from build123d import *

# Parameters (mm, degrees)
BOSS_EXTRUDE1_DEPTH = 2
CUT_EXTRUDE2_DEPTH  = 2
SKETCH5_R           = 2.25
CUT_EXTRUDE4_DEPTH  = 2


with BuildPart() as part:
    # Sketch1 → Boss-Extrude1 (new body)
    with BuildSketch(Plane(origin=(0, 0, 0), x_dir=(1, 0, 0), z_dir=(0, 1, 0))):
        Polygon((-14, -27.5), (-9, -27.5), (-9, -29.5), (-5, -29.5), (-5, -27.5), (5, -27.5), (5, -29.5), (9, -29.5), (9, -27.5), (14, -27.5), (14, 27.5), (9, 27.5), (9, 29.5), (5, 29.5), (5, 27.5), (-5, 27.5), (-5, 29.5), (-9, 29.5), (-9, 27.5), (-14, 27.5), (-14, 14.5), (-14, -14.5), align=None)
    extrude(amount=BOSS_EXTRUDE1_DEPTH)

    # Sketch4 → Cut-Extrude2 (cut)
    with BuildSketch(Plane(origin=(0, 2, 0), x_dir=(1, 0, 0), z_dir=(0, 1, 0))):
        Polygon((-1.5, 23.2), (-2.6, 23.2), (-2.6, 25.5), (-1.5, 25.5), (-1.5, 27.5), (1.5, 27.5), (1.5, 25.5), (2.6, 25.5), (2.6, 23.2), (1.5, 23.2), (1.5, 21.5), (-1.5, 21.5), align=None)
        Polygon((1.5, -25.5), (1.5, -27.5), (-1.5, -27.5), (-1.5, -25.5), (-2.6, -25.5), (-2.6, -23.2), (-1.5, -23.2), (-1.5, -21.5), (1.5, -21.5), (1.5, -23.2), (2.6, -23.2), (2.6, -25.5), align=None)
    extrude(amount=-CUT_EXTRUDE2_DEPTH, mode=Mode.SUBTRACT)

    # Sketch5 → Cut-Extrude4 (cut)
    with BuildSketch(Plane(origin=(0, 2, 0), x_dir=(1, 0, 0), z_dir=(0, 1, 0))):
        with Locations(Location((0, -9.51, 0), (0, 0, 270))):
            Circle(SKETCH5_R)
    extrude(amount=-CUT_EXTRUDE4_DEPTH, mode=Mode.SUBTRACT)


solid = part.part
Could you check a few things on this model? Use its own coordinates, in mm. A direction names the side the tool comes from. Give positions to 0.01 mm unless a question says otherwise; leave off trailing zeros. Write each loop counter-clockwise with the first axis right and the second up, starting at its lowest first coordinate (ties: lowest second). Pieces come first, ordered by that corner, then holes. Notation, with made-up numbers: (35, 20) - (75, 20) arc R23 cw to (75, 38) - close; hole circle Ø6 at (-15, 84). An arc over 180 degrees is marked (long way). Use CSV: the item, a comma, the result in double quotes. Start each with the question number.
Item 1: I want a section at A-A, the plane z = 9.51. Please give me the cut outline in (x, y), then the cut area to 3 significant figures.
Item 2: If we mould it in two halves opening along Z, with no side actions, what happens to faces 5 (the face through (0, 1, -21.5)), 6 (the face through (11, 1, 27.5)), 7 (the face through (0, 0, 0)), 8 (the face through (2, 1, -23.2))? For each: pulls with the +Z half, pulls with the -Z half, needs draft (parallel to the pull), parting line crosses it, or undercut.
Item 3: For faces 1 (the face through (-2.6, 1, 24)), 2 (the face through (-11, 1, -27.5)), 3 (the face through (-1.5, 1, -26)), 4 (the face through (1.5, 1, 22)), which set-ups out of +Z, -Z, +X, -X, +Y, -Y let a thin tool reach every point of the face, with its end or its side?
Item 4: I want a section at C-C, the plane x = -3.25. Please give me the cut outline in (y, z), then the cut area to 3 significant figures.
Item 5: If I drill on line 1 along X through (y, z) = (1.4, 27); line 2 along X through (y, z) = (0.9, 9.51); line 3 along Z through (x, y) = (-10.5, 0.95), over which ranges is the centre line in solid material (lowest first)?
Item 6: I want a section at B-B, the plane x = 0. Please give me the cut outline in (y, z).
Item 7: I'm going to push flat-ended pins straight in: pin 1 (7 mm diameter, centred on x = 0, z = 9.51, fed in from -Y); pin 2 (0.6 mm diameter, centred on x = 3, y = 0.5, fed in from +Z); pin 3 (1 mm diameter, centred on y = 1, z = 29, fed in from -X); pin 4 (1 mm diameter, centred on x = 0, y = 0.5, fed in from +Z). Where does each tip first touch, or does it pass through?
Findings:
1,outline,"(-14, 0) - (-2.25, 0) - (-2.25, 2) - (-14, 2) - close; (2.25, 0) - (14, 0) - (14, 2) - (2.25, 2) - close"
1,area,"47.0 mm2"
2,face 5,"pulls with the -Z half"
2,face 6,"pulls with the +Z half"
2,face 7,"needs draft"
2,face 8,"undercut"
3,face 1,"+Y, -Y"
3,face 2,"-Z, -X, +Y, -Y"
3,face 3,"-Z, +Y, -Y"
3,face 4,"+Z, +Y, -Y"
4,outline,"(0, -27.5) - (2, -27.5) - (2, 27.5) - (0, 27.5) - close"
4,area,"110 mm2"
5,line 1,"x = -14 to -1.5, 1.5 to 14"
5,line 2,"x = -14 to -2.25, 2.25 to 14"
5,line 3,"z = -27.5 to 27.5"
6,outline,"(0, -21.5) - (2, -21.5) - (2, 7.26) - (0, 7.26) - close; (0, 11.76) - (2, 11.76) - (2, 21.5) - (0, 21.5) - close"
7,pin 1,"stops at y = 0"
7,pin 2,"stops at z = 27.5"
7,pin 3,"stops at x = -9"
7,pin 4,"stops at z = 21.5"
